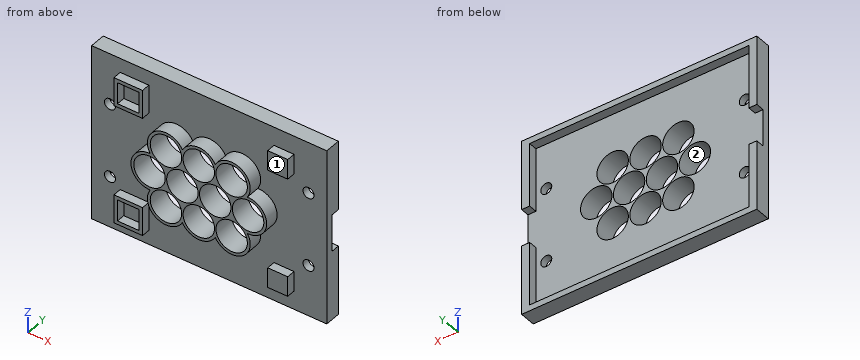
Autodesk Inventor part; units mm, degrees
ref_plane "YZ Plane" through (0, 0, 0) normal (1, 0, 0) x (0, 1, 0)
ref_plane "XZ Plane" through (0, 0, 0) normal (0, 1, 0) x (-1, 0, 0)
ref_plane "XY Plane" through (0, 0, 0) normal (0, 0, 1) x (1, 0, 0)
sketch "Sketch1" plane through (0, 0, 0) normal (0, 1, 0) x (-1, 0, 0)
  circle A0 centre (0, 0) radius 11
  line L0 (11, 0.0002) -> (12, 0.0002) construction
  circle A1 centre (23, 0) radius 11
  line L1 (34, 0) -> (35, 0) construction
  circle A2 centre (46, 0) radius 11
  line L2 (57, 0) -> (58, 0) construction
  circle A3 centre (69, 0) radius 11
  line L3 (34.5, 0) -> (34.5, -17.154) construction
  line L4 (34.5, 0) -> (34.5, 17.658) construction
  line L5 (55, 12.6387) -> (55, -13.5831) construction
  line L6 (55, 12.6387) -> (55, 17.658) construction
  line L7 (55, -13.5831) -> (55, -17.154) construction
  line L8 (11.5, 0.0002) -> (11.5, -16.2579) construction
  line L9 (11.5, 0.0002) -> (11.5, 19.9186) construction
  circle A4 centre (0, 0) radius 12 construction
  circle A5 centre (23, 0) radius 12 construction
  circle A6 centre (46, 0) radius 12 construction
  circle A7 centre (69, 0) radius 12 construction
  circle A8 centre (11.5, 19.9186) radius 11
  circle A9 centre (34.5, 19.9186) radius 11
  circle A10 centre (11.5, -19.9186) radius 11
  circle A11 centre (57.5, 19.9186) radius 11
  circle A12 centre (57.5, -19.9186) radius 12 construction
  circle A13 centre (34.5, -19.9186) radius 12 construction
  circle A14 centre (11.5, 19.9186) radius 12 construction
  circle A15 centre (34.5, 19.9186) radius 12 construction
  circle A16 centre (57.5, 19.9186) radius 12 construction
  line L10 (11.5, 19.9186) -> (57.5, 19.9186) construction
  arc A17 (2.3131, -12.7926) -> (0.5, -12.9904) centre (0, 0) ccw construction
  circle A18 centre (11.5, 19.9186) radius 13 construction
  circle A19 centre (34.5, 19.9186) radius 13 construction
  circle A20 centre (57.5, 19.9186) radius 13 construction
  circle A21 centre (69, 0) radius 13 construction
  circle A22 centre (57.5, -19.9186) radius 13 construction
  circle A23 centre (34.5, -19.9186) radius 13 construction
  arc A24 (0.5, 12.9904) -> (0.5, -12.9904) centre (0, 0) ccw
  line L11 (57.5, -19.9186) -> (11.5, -19.9186) construction
  circle A25 centre (11.5, -19.9186) radius 13 construction
  arc A26 (0.5, -12.9904) -> (23, -25.9808) centre (11.5, -19.9186) ccw
  arc A27 (23, -25.9808) -> (46, -25.9808) centre (34.5, -19.9186) ccw
  arc A28 (46, -25.9808) -> (68.5, -12.9904) centre (57.5, -19.9186) ccw
  arc A29 (68.5, -12.9904) -> (68.5, 12.9904) centre (69, 0) ccw
  arc A30 (68.5, 12.9904) -> (46, 25.9808) centre (57.5, 19.9186) ccw
  arc A31 (46, 25.9808) -> (23, 25.9808) centre (34.5, 19.9186) ccw
  arc A32 (23, 25.9808) -> (0.5, 12.9904) centre (11.5, 19.9186) ccw
  circle A33 centre (11.5, -19.9186) radius 12 construction
  circle A34 centre (34.5, -19.9186) radius 11
  circle A35 centre (57.5, -19.9186) radius 11
  dimension "d0" = 22
  dimension "d6" = 22
  dimension "d1" = 1
  dimension "d2" = 22
  dimension "d3" = 1
  dimension "d4" = 22
  dimension "d5" = 1
  dimension "d7" = 24
  dimension "d8" = 24
  dimension "d9" = 24
  dimension "d10" = 24
  dimension "d11" = 22
  dimension "d12" = 22
  dimension "d16" = 22
  dimension "d17" = 22
  dimension "d19" = 24
  dimension "d21" = 24
  dimension "d22" = 24
  dimension "d23" = 24
  dimension "d25" = 26
  dimension "d27" = 26
  dimension "d28" = 26
  dimension "d29" = 26
  dimension "d30" = 26
  dimension "d31" = 26
  dimension "d32" = 26
  dimension "d33" = 26
  dimension "d67" = 24
  dimension "d71" = 24
  dimension "d72" = 22
  dimension "d73" = 22
extrude "Extrusion1" add sketch "Sketch1" along normal blind 15
sketch "Sketch2" plane through (0, 15, 0) normal (0, 1, 0) x (1, 0, 0)
  circle A0 centre (-23, 0) radius 11
  circle A1 centre (-46, 0) radius 11
  line L0 (-35, 0) -> (-34, 0) construction
  line L1 (-111.2, 57.65) -> (42.2, 57.65)
  line L2 (42.2, 57.65) -> (42.2, -57.65)
  line L3 (42.2, -57.65) -> (-111.2, -57.65)
  line L4 (-111.2, -57.65) -> (-111.2, 57.65)
  line L5 (-111.2, 57.65) -> (42.2, -57.65) construction
  line L6 (42.2, 57.65) -> (-111.2, -57.65) construction
  arc A2 (-46, 25.9808) -> (-68.5, 12.9904) centre (-57.5, 19.9186) ccw
  arc A3 (-23, 25.9808) -> (-46, 25.9808) centre (-34.5, 19.9186) ccw
  arc A4 (-0.5, 12.9904) -> (-23, 25.9808) centre (-11.5, 19.9186) ccw
  arc A5 (-0.5, -12.9904) -> (-0.5, 12.9904) centre (0, 0) ccw
  arc A6 (-23, -25.9808) -> (-0.5, -12.9904) centre (-11.5, -19.9186) ccw
  arc A7 (-46, -25.9808) -> (-23, -25.9808) centre (-34.5, -19.9186) ccw
  arc A8 (-68.5, -12.9904) -> (-46, -25.9808) centre (-57.5, -19.9186) ccw
  arc A9 (-68.5, 12.9904) -> (-68.5, -12.9904) centre (-69, 0) ccw
  arc A10 (-69, 13) -> (-68.5, -12.9904) centre (-69, 0) ccw
  arc A11 (-46, 25.9808) -> (-68.5, 12.9904) centre (-57.5, 19.9186) ccw
  arc A12 (-23, 25.9808) -> (-46, 25.9808) centre (-34.5, 19.9186) ccw
  arc A13 (-0.5, 12.9904) -> (-23, 25.9808) centre (-11.5, 19.9186) ccw
  arc A14 (-0.5, -12.9904) -> (-0.5, 12.9904) centre (0, 0) ccw
  arc A15 (-23, -25.9808) -> (-0.5, -12.9904) centre (-11.5, -19.9186) ccw
  arc A16 (-46, -25.9808) -> (-23, -25.9808) centre (-34.5, -19.9186) ccw
  arc A17 (-68.5, -12.9904) -> (-46, -25.9808) centre (-57.5, -19.9186) ccw
  arc A18 (-68.5, 12.9904) -> (-68.5, -12.9904) centre (-69, 0) ccw
  point P0 (-34.5, 0)
  dimension "d36" = 115.3
  dimension "d37" = 153.4
extrude "Extrusion2" add sketch "Sketch2" against normal blind 5 contours L1 L2 L3 L4
sketch "Sketch3" plane through (0, 15, 0) normal (0, 1, 0) x (1, 0, 0)
  line L0 (42.2, 57.65) -> (-111.2, 57.65)
  line L1 (42.2, -57.65) -> (42.2, 57.65)
  line L2 (-111.2, -57.65) -> (42.2, -57.65)
  line L3 (-111.2, 57.65) -> (-111.2, -57.65)
  line L4 (-111.2, -57.65) -> (42.2, -57.65)
  line L5 (42.2, -57.65) -> (42.2, 57.65)
  line L6 (42.2, 57.65) -> (-111.2, 57.65)
  line L7 (-111.2, 57.65) -> (-111.2, -57.65)
  circle A0 centre (-57.5, -19.9186) radius 11
  circle A1 centre (-11.5, 19.9186) radius 11
  circle A2 centre (-34.5, -19.9186) radius 11
  circle A3 centre (-11.5, -19.9186) radius 11
  circle A4 centre (-69, 0) radius 11
  circle A5 centre (-46, 0) radius 11
  circle A6 centre (-23, 0) radius 11
  circle A7 centre (0, 0) radius 11
  line L8 (-116.8026, 61.8611) -> (47.8026, 61.8611)
  line L9 (47.8026, 61.8611) -> (47.8026, -61.8611)
  line L10 (47.8026, -61.8611) -> (-116.8026, -61.8611)
  line L11 (-116.8026, -61.8611) -> (-116.8026, 61.8611)
  line L12 (-116.8026, 61.8611) -> (47.8026, -61.8611) construction
  line L13 (47.8026, 61.8611) -> (-116.8026, -61.8611) construction
  line L14 (-111.2, -57.65) -> (42.2, -57.65)
  line L15 (42.2, -57.65) -> (42.2, 57.65)
  line L16 (42.2, 57.65) -> (-111.2, 57.65)
  line L17 (-111.2, 57.65) -> (-111.2, -57.65)
  line L18 (-111.2, -57.65) -> (42.2, 57.65) construction
  line L19 (42.2, -57.65) -> (-111.2, 57.65) construction
  point P0 (-34.5, 0)
extrude "Extrusion3" add sketch "Sketch3" along normal blind 6 and the other way blind 5 contours L8 L9 L10 L11
sketch "Sketch4" plane through (0, 15, 0) normal (0, 1, 0) x (1, 0, 0)
  line L0 (-111.2, -57.65) -> (42.2, -57.65)
  line L1 (42.2, -57.65) -> (42.2, 57.65)
  line L2 (42.2, 57.65) -> (-111.2, 57.65)
  line L3 (-111.2, 57.65) -> (-111.2, -57.65)
  circle A0 centre (-57.5, -19.9186) radius 11
  circle A1 centre (-11.5, 19.9186) radius 11
  circle A2 centre (-34.5, -19.9186) radius 11
  circle A3 centre (-11.5, -19.9186) radius 11
  circle A4 centre (-69, 0) radius 11
  circle A5 centre (-46, 0) radius 11
  circle A6 centre (-23, 0) radius 11
  circle A7 centre (0, 0) radius 11
  line L4 (-111.2, 57.65) -> (-103.972, 57.65) construction
  line L5 (-103.972, 57.65) -> (-103.972, 25.9) construction
  line L6 (-103.972, 25.9) -> (-111.2, 25.9) construction
  line L7 (-111.2, 25.9) -> (-111.2, 57.65) construction
  line L8 (42.2, 57.65) -> (34.972, 57.65) construction
  line L9 (34.972, 57.65) -> (34.972, 25.9) construction
  line L10 (34.972, 25.9) -> (42.2, 25.9) construction
  line L11 (42.2, 25.9) -> (42.2, 57.65) construction
  line L12 (-111.2, -57.65) -> (-103.972, -57.65) construction
  line L13 (-103.972, -57.65) -> (-103.972, -25.9) construction
  line L14 (-103.972, -25.9) -> (-111.2, -25.9) construction
  line L15 (-111.2, -25.9) -> (-111.2, -57.65) construction
  line L16 (42.2, -25.9) -> (34.972, -25.9) construction
  line L17 (34.972, -25.9) -> (34.972, -57.65) construction
  line L18 (34.972, -57.65) -> (42.2, -57.65) construction
  line L19 (42.2, -57.65) -> (42.2, -25.9) construction
  circle A8 centre (-103.972, 25.9) radius 3.865
  circle A9 centre (34.972, 25.9) radius 3.865
  circle A10 centre (34.972, -25.9) radius 3.865
  circle A11 centre (-103.972, -25.9) radius 3.865
  dimension "d56" = 7.73
  dimension "d57" = 7.73
  dimension "d58" = 7.73
  dimension "d59" = 7.73
  dimension "d62" = 7.228
  dimension "d63" = 31.75
  dimension "d64" = 7.228
  dimension "d65" = 7.228
  dimension "d66" = 31.75
extrude "Extrusion4" cut sketch "Sketch4" against normal through all contours A8 | A9 | A10 | A11
sketch "Sketch5" plane through (-116.8026, 10, 61.8611) normal (-1, 0, 0) x (0, 0, 1)
  line L0 (-74.8611, -12) -> (-74.8611, -2)
  line L1 (-48.8611, -12) -> (-48.8611, -2)
  line L2 (-119.5111, 5) -> (-4.2111, 5)
  line L3 (-123.7222, 11) -> (0, 11)
  line L4 (-74.8611, 5) -> (-48.8611, 5)
  line L5 (-48.8611, 5) -> (-48.8611, 11)
  line L6 (-48.8611, 11) -> (-74.8611, 11)
  line L7 (-74.8611, 11) -> (-74.8611, 5)
  point P0 (-61.8611, -10)
  point P1 (-74.8611, 11)
extrude "Extrusion5" cut sketch "Sketch5" against normal through all
sketch "Sketch6" plane through (0, 10, 0) normal (0, -1, 0) x (1, 0, 0)
  circle A0 centre (34.972, 25.9) radius 3.865
  circle A1 centre (34.972, -25.9) radius 3.865
  circle A2 centre (-103.972, 25.9) radius 3.865
  circle A3 centre (-103.972, -25.9) radius 3.865
  line L0 (47.8026, 61.8611) -> (-116.8026, 61.8611)
  line L1 (-116.8026, 61.8611) -> (-116.8026, -61.8611)
  line L2 (-116.8026, -61.8611) -> (47.8026, -61.8611)
  line L3 (47.8026, -61.8611) -> (47.8026, 61.8611)
  arc A4 (-68.5, 12.9904) -> (-68.5, -12.9904) centre (-69, 0) ccw
  arc A5 (-46, 25.9808) -> (-68.5, 12.9904) centre (-57.5, 19.9186) ccw
  arc A6 (-23, 25.9808) -> (-46, 25.9808) centre (-34.5, 19.9186) ccw
  arc A7 (-0.5, 12.9904) -> (-23, 25.9808) centre (-11.5, 19.9186) ccw
  arc A8 (-0.5, -12.9904) -> (-0.5, 12.9904) centre (0, 0) ccw
  arc A9 (-23, -25.9808) -> (-0.5, -12.9904) centre (-11.5, -19.9186) ccw
  arc A10 (-46, -25.9808) -> (-23, -25.9808) centre (-34.5, -19.9186) ccw
  arc A11 (-68.5, -12.9904) -> (-46, -25.9808) centre (-57.5, -19.9186) ccw
  line L4 (-116.8026, 61.8611) -> (-86.8026, 61.8611) construction
  line L5 (-86.8026, 61.8611) -> (-116.8026, 61.8611) construction
  line L6 (-116.8026, 61.8611) -> (-116.8026, 41.8611) construction
  line L7 (-96.8026, 51.8611) -> (-76.8026, 51.8611)
  line L8 (-76.8026, 51.8611) -> (-76.8026, 31.8611)
  line L9 (-76.8026, 31.8611) -> (-96.8026, 31.8611)
  line L10 (-96.8026, 31.8611) -> (-96.8026, 51.8611)
  line L11 (-96.8026, 51.8611) -> (-76.8026, 31.8611) construction
  line L12 (-76.8026, 51.8611) -> (-96.8026, 31.8611) construction
  line L13 (-94.3026, 49.3611) -> (-79.3026, 49.3611)
  line L14 (-79.3026, 49.3611) -> (-79.3026, 34.3611)
  line L15 (-79.3026, 34.3611) -> (-94.3026, 34.3611)
  line L16 (-94.3026, 34.3611) -> (-94.3026, 49.3611)
  line L17 (-94.3026, 49.3611) -> (-79.3026, 34.3611) construction
  line L18 (-79.3026, 49.3611) -> (-94.3026, 34.3611) construction
  line L19 (-116.8026, 0) -> (47.8026, 0) construction
  line L20 (-96.8026, -51.8611) -> (-76.8026, -51.8611)
  line L21 (-76.8026, -51.8611) -> (-76.8026, -31.8611)
  line L22 (-76.8026, -31.8611) -> (-96.8026, -31.8611)
  line L23 (-96.8026, -31.8611) -> (-96.8026, -51.8611)
  line L24 (-96.8026, -51.8611) -> (-76.8026, -31.8611) construction
  line L25 (-76.8026, -51.8611) -> (-96.8026, -31.8611) construction
  line L26 (-94.3026, -49.3611) -> (-79.3026, -49.3611)
  line L27 (-79.3026, -49.3611) -> (-79.3026, -34.3611)
  line L28 (-79.3026, -34.3611) -> (-94.3026, -34.3611)
  line L29 (-94.3026, -34.3611) -> (-94.3026, -49.3611)
  line L30 (-94.3026, -49.3611) -> (-79.3026, -34.3611) construction
  line L31 (-79.3026, -49.3611) -> (-94.3026, -34.3611) construction
  line L32 (47.8026, 61.8611) -> (17.8026, 61.8611) construction
  line L33 (47.8026, 61.8611) -> (47.8026, 41.8611) construction
  line L34 (10.8026, 48.8611) -> (24.8026, 48.8611)
  line L35 (24.8026, 48.8611) -> (24.8026, 34.8611)
  line L36 (24.8026, 34.8611) -> (10.8026, 34.8611)
  line L37 (10.8026, 34.8611) -> (10.8026, 48.8611)
  line L38 (10.8026, 48.8611) -> (24.8026, 34.8611) construction
  line L39 (24.8026, 48.8611) -> (10.8026, 34.8611) construction
  line L40 (10.8026, -48.8611) -> (24.8026, -48.8611)
  line L41 (24.8026, -48.8611) -> (24.8026, -34.8611)
  line L42 (24.8026, -34.8611) -> (10.8026, -34.8611)
  line L43 (10.8026, -34.8611) -> (10.8026, -48.8611)
  line L44 (10.8026, -48.8611) -> (24.8026, -34.8611) construction
  line L45 (24.8026, -48.8611) -> (10.8026, -34.8611) construction
  point P0 (-86.8026, 41.8611)
  point P1 (-86.8026, 41.8611)
  point P2 (-86.8026, -41.8611)
  point P3 (-86.8026, -41.8611)
  point P4 (17.8026, 41.8611)
  point P5 (17.8026, -41.8611)
  dimension "d76" = 30
  dimension "d77" = 20
  dimension "d78" = 20
  dimension "d79" = 20
  dimension "d80" = 15
  dimension "d81" = 15
  dimension "d82" = 30
  dimension "d83" = 20
  dimension "d84" = 14
  dimension "d85" = 14
extrude "Extrusion6" add sketch "Sketch6" along normal blind 6 contours L7 L8 L9 L10 | L23 L22 L21 L20 | L34 L35 L36 L37 | L43 L42 L41 L40
properties part number "CELLCASE21700_3DPrint"
Part model, mm, in its own coordinate system. Face numbers are marked on the shaded views. Round coordinates to 2 decimals unless told otherwise and drop trailing zeros. Write each loop counter-clockwise with the first axis right and the second up, starting at its lowest first coordinate (ties: lowest second). Pieces come first, ordered by that corner, then holes. Notation, with made-up numbers: M 73.25,84.25 L 131.25,84.25 A20 cw 131.25,113.25 Z; hole C 40.5,36.25 d4. An arc over 180 degrees is marked long. Answer as CSV lines item,"result". Start each with the question number.
1) Band-saw the part on B-B (z = 0). List the corners of the cut face in (x, y).
2) Band-saw the part on A-A (y = 19.25). List the corners of the cut face in (x, z).
3) Drill centre lines: L1, parallel to X at y = 9.5, z = 37; L2, parallel to Z at x = -57.5, y = 4; L3, parallel to Z at x = -80, y = 15.75. Where is each one in solid material? Low to high.
4) Band-saw the part on C-C (z = -18). List the corners of the cut face in (x, y).
5) Band-saw the part on D-D (x = -14.5). List the corners of the cut face in (y, z).
6) Drop flat-ended pins along their axis: pin 1 (5 mm diameter, centred on x = -88, y = 7, fed in from +Z); pin 2 (12 mm diameter, centred on y = 5.5, z = 41, fed in from +X); pin 3 (4.5 mm diameter, centred on x = -89.5, z = -42.5, fed in from -Y); pin 4 (5 mm diameter, centred on y = 7, z = 38.5, fed in from +X). Give the stop position or say it passes through.
7) Mould opens along Z. For the marked faces 1 and 2 say: +Z half, -Z half, draft (parallel to the pull), parting line (faces both ways), or undercut.
Worked out:
1,outline,"M -116.8,10 L -82,10 L -82,0 L -80,0 L -80,15 L -116.8,15 Z; M -58,0 L -57,0 L -57,15 L -58,15 Z; M -35,0 L -34,0 L -34,15 L -35,15 Z; M -12,0 L -11,0 L -11,15 L -12,15 Z; M 11,0 L 13,0 L 13,10 L 47.8,10 L 47.8,15 L 11,15 Z"
2,outline,"M -116.8,-61.86 L 47.8,-61.86 L 47.8,-13 L 42.2,-13 L 42.2,-57.65 L -111.2,-57.65 L -111.2,-13 L -116.8,-13 Z; M -116.8,13 L -111.2,13 L -111.2,57.65 L 42.2,57.65 L 42.2,13 L 47.8,13 L 47.8,61.86 L -116.8,61.86 Z"
3,L1,"-96.8 to -94.3, -79.3 to -76.8, 10.8 to 24.8"
3,L2,"-32.92 to -30.92, -8.92 to 8.92, 30.92 to 32.92"
3,L3,"-61.86 to -57.65, 57.65 to 61.86"
4,outline,"M -116.8,10 L -70.36,10 L -70.36,0 L -68.33,0 L -68.33,15 L -111.2,15 L -111.2,21 L -116.8,21 Z; M -46.67,0 L -45.33,0 L -45.33,15 L -46.67,15 Z; M -23.67,0 L -22.33,0 L -22.33,15 L -23.67,15 Z; M -0.67,0 L 1.36,0 L 1.36,10 L 47.8,10 L 47.8,21 L 42.2,21 L 42.2,15 L -0.67,15 Z"
5,outline,"M 0,-32.57 L 10,-32.57 L 10,-61.86 L 21,-61.86 L 21,-57.65 L 15,-57.65 L 15,-30.5 L 0,-30.5 Z; M 0,-9.34 L 15,-9.34 L 15,-6.98 L 0,-6.98 Z; M 0,6.98 L 15,6.98 L 15,9.34 L 0,9.34 Z; M 0,30.5 L 15,30.5 L 15,57.65 L 21,57.65 L 21,61.86 L 10,61.86 L 10,32.57 L 0,32.57 Z"
6,pin 1,"z = 51.86"
6,pin 2,"x = 47.8"
6,pin 3,"y = 10"
6,pin 4,"x = 24.8"
7,face 1,"draft"
7,face 2,"undercut"
